Check sheet for the modelled part. Datum: model origin and axes. Units: mm. A direction names the side the tool comes from. Round coordinates to 2 decimals unless told otherwise and drop trailing zeros. Order: outer loops, then holes, each group sorted by start corner. A loop starts at its lowest first (then second) coordinate and runs counter-clockwise, first axis right, second up.
(1) Sectioned sample at C-C, the plane z = 7.5. Enter the section's corners in (x, y).
(2) Mould release check, pull along X, two halves, no side actions. Record for faces 1 (the flat face through (-16.993, 3, 11)), 2 (the flat face through (-3.045, 3, -8)), 3 (the flat face through (-18, 3, 11.87)): released by +X, released by -X, zero draft, split by the parting line, or undercut.
(3) Depth check by flat-ended pin: pin 1 (0.8 mm diameter, centred on x = -18, y = 4, fed in from +Z); pin 2 (2 mm diameter, centred on x = -18.5, y = 3, fed in from -Z); pin 3 (0.9 mm diameter, centred on y = 3.5, z = -8.5, fed in from +X). Enter the tip coordinate at first touch or a pass-through.
(4) Tool access check on faces 4 (the flat face through (-18, 3, 10.524)), 5 (the flat face through (24, 3, -9.339)), 6 (the flat face through (-19.559, 3, 11)), 7 (the flat face through (0, 0.1, 0)). Record the directions out of +Z, -Z, +X, -X, +Y, -Y that give a thin tool (end or side, any length) a straight path to the whole face; none if there is none.
(5) Sectioned sample at B-B, the plane x = 2. Enter the section's corners in (y, z), and give its area (3 significant figures).
(6) Sectioned sample at A-A, the plane y = 3.55. Enter the section's corners in (x, z), and give its area (3 significant figures).
(7) Thickness scan on probe 1 along X at (y, z) = (2.05, -8); probe 2 along Y at (x, z) = (21.5, -22.5); probe 3 along X at (y, z) = (2, -5). Record the ranges inside material, lowest first.
```python
from build123d import *

# Parameters (mm, degrees)
BOSS_EXTRUDE1_DEPTH = 2
SCALE1_SCALE        = 0.9
SKETCH3_W           = 6.046779213
SKETCH3_H           = 4.468776405
BOSS_EXTRUDE2_DEPTH = 3
SKETCH4_W           = 2.790397576
SKETCH4_H           = 6.115363286
BOSS_EXTRUDE3_DEPTH = 3
SKETCH5_W           = 2.56611171
SKETCH5_H           = 1.346193589
BOSS_EXTRUDE4_DEPTH = 3


with BuildPart() as part:
    # Sketch2 → Boss-Extrude1 (new body)
    with BuildSketch(Plane(origin=(0, 0, 0), x_dir=(1, 0, 0), z_dir=(0, 1, 0))):
        with BuildLine():
            Line((-10, 30), (20, 30))
            ThreePointArc((20, 30), (27.071067812, 27.071067812), (30, 20))
            Line((30, 20), (30, -20))
            ThreePointArc((30, -20), (27.071067812, -27.071067812), (20, -30))
            Line((20, -30), (-20, -30))
            ThreePointArc((-20, -30), (-27.071067812, -27.071067812), (-30, -20))
            Line((-30, -20), (-30, 10))
            ThreePointArc((-30, 10), (-24.142135624, 24.142135624), (-10, 30))
        make_face()
    extrude(amount=BOSS_EXTRUDE1_DEPTH)


with BuildPart() as part_1:
    # Scale1: scaled about (0.462600785, 1, 0.462600785)
    add(part.part.scale(SCALE1_SCALE).moved(Location((0.046260078, 0.1, 0.046260078))))

    # Sketch3 → Boss-Extrude2 (add)
    with BuildSketch(Plane(origin=(0, 1.9, 0), x_dir=(1, 0, 0), z_dir=(0, 1, 0))):
        with Locations((-6.068725182, 8.270529837)):
            Rectangle(SKETCH3_W, SKETCH3_H)
    extrude(amount=BOSS_EXTRUDE2_DEPTH)

    # Sketch4 → Boss-Extrude3 (add)
    with BuildSketch(Plane(origin=(0, 1.9, 0), x_dir=(1, 0, 0), z_dir=(0, 1, 0))):
        with Locations((24.212308402, 6.281277774)):
            Rectangle(SKETCH4_W, SKETCH4_H)
    extrude(amount=BOSS_EXTRUDE3_DEPTH)

    # Sketch5 → Boss-Extrude4 (add)
    with BuildSketch(Plane(origin=(0, 1.9, 0), x_dir=(1, 0, 0), z_dir=(0, 1, 0))):
        with Locations((-18.275730646, -11.196811513)):
            Rectangle(SKETCH5_W, SKETCH5_H)
    extrude(amount=BOSS_EXTRUDE4_DEPTH)


solid = part_1.part
```
Derived:
1. outline: (-26.95, 0.1) - (27.05, 0.1) - (27.05, 1.9) - (-26.95, 1.9) - close
2. face 1: released by +X
2. face 2: undercut
2. face 3: zero draft
3. pin 1: stops at z = 11.87
3. pin 2: stops at z = 10.52
3. pin 3: stops at x = 25.61
4. face 4: -Z, +X, -X, +Y
4. face 5: -Z, +X, +Y
4. face 6: +Z, -Z, -X, +Y
4. face 7: +Z, -Z, +X, -X, -Y
5. outline: (0.1, -26.95) - (1.9, -26.95) - (1.9, 27.05) - (0.1, 27.05) - close
5. area: 97.2 mm2
6. outline: (-19.56, 10.52) - (-16.99, 10.52) - (-16.99, 11.87) - (-19.56, 11.87) - close; (-9.09, -10.5) - (-3.05, -10.5) - (-3.05, -6.04) - (-9.09, -6.04) - close; (22.82, -9.34) - (25.61, -9.34) - (25.61, -3.22) - (22.82, -3.22) - close
6. area: 47.5 mm2
7. probe 1: x = -9.09 to -3.05, 22.82 to 25.61
7. probe 2: y = 0.1 to 1.9
7. probe 3: x = 22.82 to 25.61
